For this review, use the dimensioned drawing (mm, ordinates from the lowest corner) and the shaded views. A direction names the side the tool comes from. Give positions to 0.01 mm unless a question says otherwise; leave off trailing zeros. Write each loop counter-clockwise with the first axis right and the second up, starting at its lowest first coordinate (ties: lowest second). Pieces come first, ordered by that corner, then holes. Notation, with made-up numbers: M 4,14 L 38,14 A17 cw 38,21 Z; hole C 74.5,-7 d8. An arc over 180 degrees is marked long. One line per item, written item: value. Start each with the question number.
Item 1: To check wall thickness, follow probe 1 along X at (y, z) = (20.1, 10); probe 2 along X at (y, z) = (8.25, 2.5); probe 3 along Y at (x, z) = (29.25, 10). State the ranges of each line that lie inside material, in increasing order.
Item 2: Consider section B-B, the plane z = 10. Give the number of separate pieces and of enclosed holes in the cut face, and give its area (3 significant figures).
Item 3: Clearance check with flat-ended pins moving along their axes: pin 1 Ø10 at (x, z) = (14.5, 4.5) entering from +Y; pin 2 Ø4.5 at (x, z) = (27, 10) entering from +Y. State where each tip first meets the part, or that it passes through.
Item 4: Consider section D-D, the plane x = 2.5. Write out the cut boundary in (y, z).
Item 5: Mouldability with a two-part tool opening along Y and no side actions: class the marked faces 4, 5 and 6 as released by +Y, released by -Y, zero draft, split by the parting line, or undercut.
Item 6: Tool access review of the marked faces 1, 2 and 3: name each direction out of +Z, -Z, +X, -X, +Y, -Y from which nothing blocks a thin tool from reaching the whole face with its end or side.
Item 7: Consider section A-A, the plane y = 7. Write out the cut boundary in (x, z).
Item 8: Consider section C-C, the plane y = 13. Write out the cut boundary in (x, z), and give its area (3 significant figures).
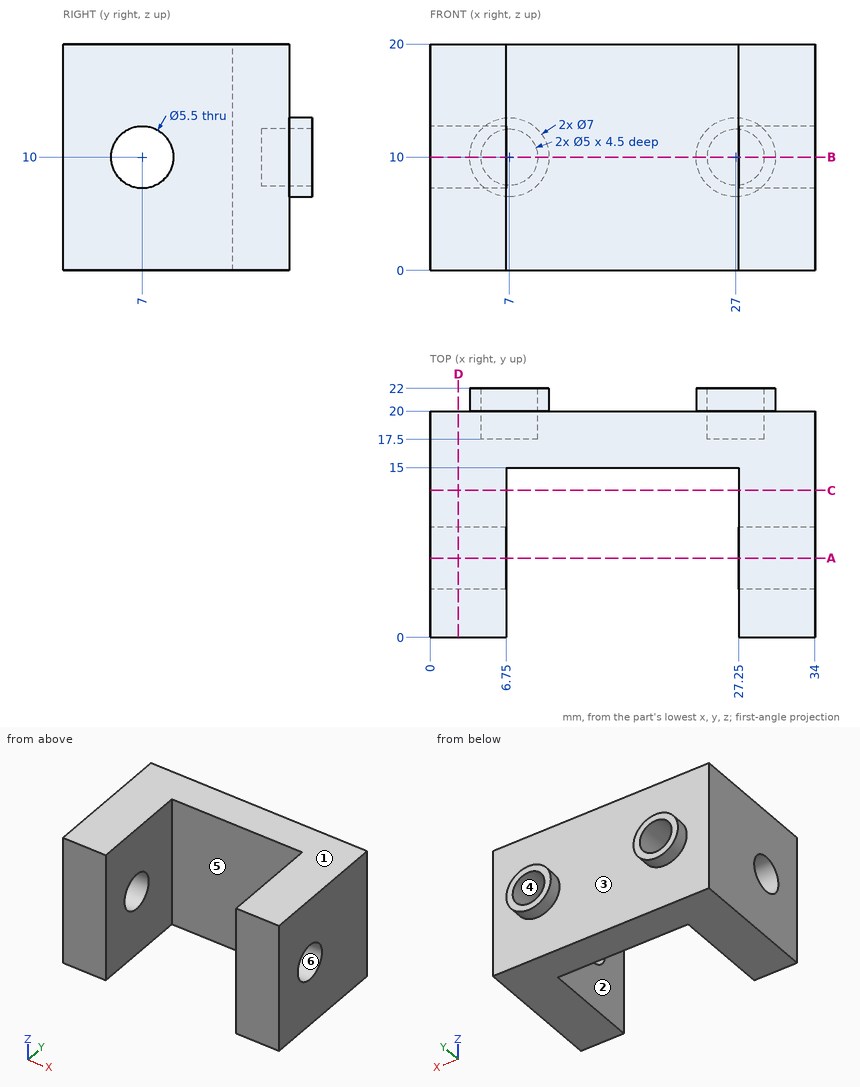
Model answer:
1. probe 1: x = 3.5 to 4.5, 9.5 to 10.5, 23.5 to 24.5, 29.5 to 30.5
1. probe 2: x = 0 to 6.75, 27.25 to 34
1. probe 3: y = 0 to 4.25, 9.75 to 17.5
2. separate pieces: 3
2. enclosed holes: 0
2. area: 281 mm2
3. pin 1: stops at y = 20
3. pin 2: stops at y = 17.5
4. outline: M 0,0 L 20,0 L 20,20 L 0,20 Z; hole C 7,10 d5.5
5. face 4: zero draft
5. face 5: released by -Y
5. face 6: undercut
6. face 1: +Z, +X, -X, +Y, -Y
6. face 2: +Z, -Z, -Y
6. face 3: +Y
7. outline: M 0,0 L 6.75,0 L 6.75,7.25 L 0,7.25 Z; M 0,12.75 L 6.75,12.75 L 6.75,20 L 0,20 Z; M 27.25,0 L 34,0 L 34,7.25 L 27.25,7.25 Z; M 27.25,12.75 L 34,12.75 L 34,20 L 27.25,20 Z
8. outline: M 0,0 L 6.75,0 L 6.75,20 L 0,20 Z; M 27.25,0 L 34,0 L 34,20 L 27.25,20 Z
8. area: 270 mm2
